Here's how the part is built. I have some questions about the finished solid (model axes, mm). Face numbers are marked on the shaded views. A direction names the side the tool comes from. Round coordinates to 2 decimals unless told otherwise and drop trailing zeros. Write each loop counter-clockwise with the first axis right and the second up, starting at its lowest first coordinate (ties: lowest second). Pieces come first, ordered by that corner, then holes. Notation, with made-up numbers: (89, 64.25) - (96, 64.25) arc R16 ccw to (96, 86.25) - close; hole circle Ø8 at (1.25, 3.25). An arc over 180 degrees is marked (long way). One line per item, written item: value. Start each with the question number.
Item 1: For the marked faces 1, 2 and 3, which set-ups out of +Z, -Z, +X, -X, +Y, -Y let a thin tool reach every point of the face, with its end or its side?
Item 2: For P1, Ø5, axis at y = 10.5, z = 5, coming from the +X side; P2, Ø12, axis at x = 0, y = 5.5, coming from the -Z side; P3, Ø2, axis at x = -2.5, z = 3.5, coming from the +Y side; P4, Ø5, axis at y = -3, z = 5, coming from the -X side, each with a flat end and sliding along its axis, tell me the tip position at first contact or that it passes through.
Item 3: Imagine slicing it at A-A, the plane y = 0. Please give me the cut outline in (x, z) (1 decimal).
Item 4: Thinking about a two-plate mould opening in Y: for the marked faces 4, 5 and 6, which applies, released by +Y, released by -Y, zero draft, split by the parting line, or undercut?
Item 5: If I drill on line 1 (Y direction, x = 0, z = 6); line 2 (Z direction, x = -14, y = 6.5); line 3 (X direction, y = -0.5, z = 0.5), over which ranges is the centre line in solid material (lowest first)?
Item 6: Imagine slicing it at D-D, the plane x = -12. Please give me the cut outline in (y, z) (3 decimals).
Item 7: Imagine slicing it at C-C, the plane z = 8.25. Please give me the cut outline in (x, y) (1 decimal).
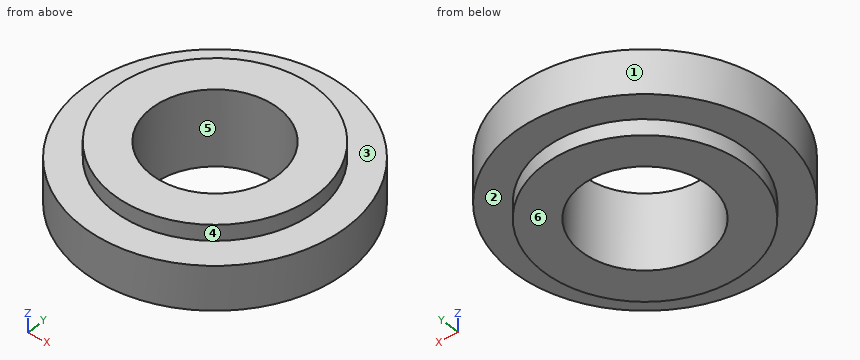
```python
from build123d import *

# Parameters (mm, degrees)
SKETCH1_R           = 12.7
SKETCH1_R_2         = 7.9375
BOSS_EXTRUDE1_DEPTH = 9.525
SKETCH2_R           = 16.51
SKETCH2_R_2         = 7.9375
BOSS_EXTRUDE2_DEPTH = 2.778125


with BuildPart() as part:
    # Sketch1 → Boss-Extrude1 (new body)
    with BuildSketch(Plane.XY):
        with Locations(Location((0, 0, 0), (0, 0, 180))):
            Circle(SKETCH1_R)
        with Locations(Location((0, 0, 0), (0, 0, 180))):
            Circle(SKETCH1_R_2, mode=Mode.SUBTRACT)
    extrude(amount=BOSS_EXTRUDE1_DEPTH)

    # Sketch2 → Boss-Extrude2 (add, symmetric)
    with BuildSketch(Plane.XY.offset(4.7625)):
        Circle(SKETCH2_R)
        with Locations(Location((0, 0, 0), (0, 0, 180))):
            Circle(SKETCH2_R_2, mode=Mode.SUBTRACT)
    extrude(amount=BOSS_EXTRUDE2_DEPTH, both=True)


solid = part.part
```
Values follow:
1. face 1: +Z, -Z
1. face 2: -Z
1. face 3: +Z
2. P1: stops at x = 14.44
2. P2: stops at z = 0
2. P3: stops at y = 16.44
2. P4: stops at x = -16.5
3. outline: (-16.5, 2) - (-12.7, 2) - (-12.7, 0) - (-7.9, 0) - (-7.9, 9.5) - (-12.7, 9.5) - (-12.7, 7.5) - (-16.5, 7.5) - close; (7.9, 0) - (12.7, 0) - (12.7, 2) - (16.5, 2) - (16.5, 7.5) - (12.7, 7.5) - (12.7, 9.5) - (7.9, 9.5) - close
4. face 4: split by the parting line
4. face 5: undercut
4. face 6: zero draft
5. line 1: y = -16.51 to -7.94, 7.94 to 16.51
5. line 2: z = 1.98 to 7.54
5. line 3: x = -12.69 to -7.92, 7.92 to 12.69
6. outline: (-11.339, 1.984) - (-4.158, 1.984) - (-4.158, 0) - (4.158, 0) - (4.158, 1.984) - (11.339, 1.984) - (11.339, 7.541) - (4.158, 7.541) - (4.158, 9.525) - (-4.158, 9.525) - (-4.158, 7.541) - (-11.339, 7.541) - close
7. outline: circle Ø25.4 at (0, 0); hole circle Ø15.9 at (0, 0)
